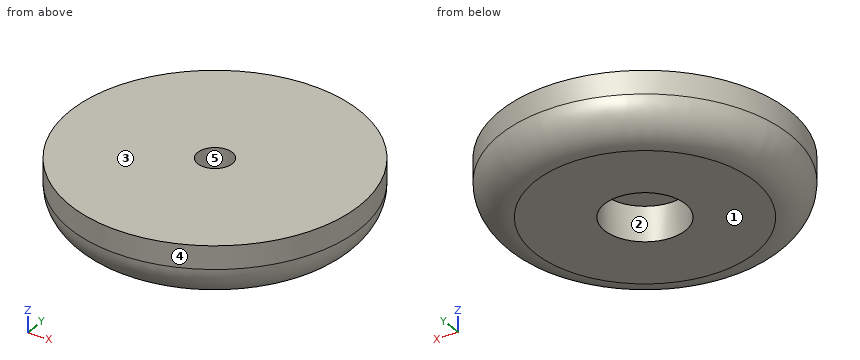
from build123d import *

# Parameters (mm, degrees)
F5_R           = 12.5
F6_DEPTH       = 5
F7_D           = 3
F7_CBORE_D     = 7
F7_CBORE_DEPTH = 3
F8_R           = 3


with BuildPart() as f6:
    # F5 (on Top) → F6 (new body)
    with BuildSketch(Plane.XY):
        Circle(F5_R)
    extrude(amount=F6_DEPTH)

    # F7 (through all)
    with Locations(Plane(origin=(0, 0, 0), x_dir=(1, 0, 0), z_dir=(0, 0, -1))):
        with Locations((0, 0)):
            CounterBoreHole(F7_D / 2, F7_CBORE_D / 2, F7_CBORE_DEPTH)

    # F8
    f8_edges = [f6.edges().sort_by_distance(p)[0] for p in [
        (-12.5, 0, 0),
    ]]
    fillet(f8_edges, radius=F8_R)


solid = f6.part
Input: part model. Units: mm. Frame: model coordinates. Face numbers are marked on the shaded views. A direction names the side the tool comes from. Coordinates: 2 decimals unless noted, no trailing zeros. Loops run counter-clockwise (first coordinate to the right, second up) from the corner with the lowest first, then second, coordinate; pieces in that order, holes last.
Q1. Material intervals for line 1 (Y direction, x = 0, z = 4.6); line 2 (X direction, y = 2, z = 2.8); line 3 (Y direction, x = 0, z = 1.15), sorted ascending.
Q2. Cut plane A-A (y = 0). Output: boundary loops of the cut face in (x, z).
Q3. Contact query for flat-ended pins moving along their axis: pin 1 (2 mm diameter, centred on y = 9, z = 3.5, fed in from +X); pin 2 (1.5 mm diameter, centred on y = 9.5, z = 1.5, fed in from +X); pin 3 (2 mm diameter, centred on x = -4.5, z = 3.5, fed in from +Y). Output: stop coordinate, or through.
Q4. Set-up query: the marked faces 1 and 2. Return all of +Z, -Z, +X, -X, +Y, -Y with unobstructed straight access to the full face (end or side cutting, diameter ignored); none if empty.
Q5. Cut plane D-D (z = 2.15). Output: boundary loops of the cut face in (x, y), then the cut area to 3 significant figures.
Q6. Cut plane C-C (z = 3.45). Output: boundary loops of the cut face in (x, y), then the cut area to 3 significant figures.
Q7. Draft query along X for the marked faces 3, 4 and 5. Return one class per face: +X half, -X half, draft (parallel to the pull), parting line (faces both ways), or undercut.
Working result:
1. line 1: y = -12.5 to -1.5, 1.5 to 12.5
1. line 2: x = -12.33 to -2.87, 2.87 to 12.33
1. line 3: y = -11.86 to -3.5, 3.5 to 11.86
2. outline: (-12.5, 3) arc R3 ccw to (-9.5, 0) - (-3.5, 0) - (-3.5, 3) - (-1.5, 3) - (-1.5, 5) - (-12.5, 5) - close; (1.5, 3) - (3.5, 3) - (3.5, 0) - (9.5, 0) arc R3 ccw to (12.5, 3) - (12.5, 5) - (1.5, 5) - close
3. pin 1: stops at x = 9.6
3. pin 2: stops at x = 8.51
3. pin 3: stops at y = 12
4. face 1: -Z, +X, -X, +Y, -Y
4. face 2: -Z
5. outline: circle Ø24.75 at (0, 0); hole circle Ø7 at (0, 0)
5. area: 443 mm2
6. outline: circle Ø25 at (0, 0); hole circle Ø3 at (0, 0)
6. area: 484 mm2
7. face 3: draft
7. face 4: parting line
7. face 5: undercut
